Work out the finished part from the listing and answer in its coordinate system (mm). A direction names the side the tool comes from. Coordinates: 2 decimals unless noted, no trailing zeros. Order: outer loops, then holes, each group sorted by start corner. A loop starts at its lowest first (then second) coordinate and runs counter-clockwise, first axis right, second up.
1. A tool of negligible diameter and unlimited length cuts with its end or side. For faces 1 (the flat face through (-5, 0, 10)), 2 (the flat face through (-5, 3, -5)), from which of +Z, -Z, +X, -X, +Y, -Y can it reach the whole face along a straight path? Write none if from no direction.
2. Flat-ended cylindrical pins translate along their axes: pin 1 Ø8 at (x, y) = (-5, -168) entering from -Z; pin 2 Ø5 at (x, y) = (10.5, 109.5) entering from +Z. Find the tip coordinate at first contact, or state that the pin passes through.
3. The part is cut by section A-A, the plane y = -59.5. Give the vertices of the cut face in (x, z), then the cut area to 3 significant figures.
4. Find the intervals of material crossed by probe 1 along Z at (x, y) = (2, -154); probe 2 along X at (y, z) = (-63.5, 0); probe 3 along Z at (x, y) = (6, 70.5), in increasing order.
5. Determine the mould class of faces 3 (the cylindrical face through (-25, 0, 0)), 4 (the flat face through (-5, -200, 7)), 5 (the flat face through (-5, 3, 5)) for opening direction X: +X half, -X half, draft (parallel to the pull), parting line (faces both ways), or undercut.
```python
from build123d import *

# Parameters (mm, degrees)
BOSS_EXTRUDE1_DEPTH = 200
SKETCH2_R           = 3
CUT_EXTRUDE1_DEPTH  = 203.546291005
FILLET1_R           = 5


with BuildPart() as part:
    # Sketch1 → Boss-Extrude1 (new, symmetric)
    with BuildSketch(Plane(origin=(0, 0, 0), x_dir=(1, 0, 0), z_dir=(0, 1, 0))):
        with BuildLine():
            Line((-15, 10), (5, 10))
            ThreePointArc((5, 10), (15, 0), (5, -10))
            Line((5, -10), (-15, -10))
            ThreePointArc((-15, -10), (-25, 0), (-15, 10))
        make_face()
        with BuildLine():
            Line((-15, 5), (5, 5))
            ThreePointArc((5, 5), (10, 0), (5, -5))
            Line((5, -5), (-15, -5))
            ThreePointArc((-15, -5), (-20, 0), (-15, 5))
        make_face(mode=Mode.SUBTRACT)
    extrude(amount=BOSS_EXTRUDE1_DEPTH, both=True)

    # Sketch2 → Cut-Extrude1 (cut, through all)
    with BuildSketch(Plane.XY.offset(10)):
        with Locations((-5, -168)):
            Circle(SKETCH2_R)
    extrude(amount=-CUT_EXTRUDE1_DEPTH, mode=Mode.SUBTRACT)

    # Fillet1
    fillet1_edges = [part.edges().sort_by_distance(p)[0] for p in [
        (15, 200, 0),
        (-5, 200, -10),
        (-25, 200, 0),
        (-5, 200, 10),
    ]]
    fillet(fillet1_edges, radius=FILLET1_R - 0.0001)  # a hair under: the kernel refuses the full size


solid = part.part
```
Geometry says:
1. face 1: +Z, +X, -X, +Y, -Y
1. face 2: +Y, -Y
2. pin 1: stops at z = -10
2. pin 2: stops at z = 9.54
3. outline: (-15, -10) - (5, -10) arc R10 ccw to (5, 10) - (-15, 10) arc R10 ccw to start; hole (-15, -5) - (5, -5) arc R5 ccw to (5, 5) - (-15, 5) arc R5 ccw to start
3. area: 436 mm2
4. probe 1: z = -10 to -5, 5 to 10
4. probe 2: x = -25 to -20, 10 to 15
4. probe 3: z = -9.95 to -4.9, 4.9 to 9.95
5. face 3: -X half
5. face 4: draft
5. face 5: undercut
